The listing builds one solid part. Answer for the finished solid, in the listing's coordinates (mm). Face numbers are marked on the shaded views. A direction names the side the tool comes from. Give positions to 0.01 mm unless a question says otherwise; leave off trailing zeros. Order: outer loops, then holes, each group sorted by start corner. A loop starts at its lowest first (then second) coordinate and runs counter-clockwise, first axis right, second up. Notation, with made-up numbers: (86, 86) - (145, 86) arc R17 cw to (145, 90) - close; hole circle Ø4 at (4, 44). An arc over 180 degrees is marked (long way). Answer in a Markdown table with one row per item. Add a question column.
```python
from build123d import *

# Parameters (mm, degrees)
SKETCH3_W           = 13.5
SKETCH3_H           = 5
SKETCH3_W_2         = 10
SKETCH3_W_3         = 5
SKETCH3_H_2         = 23
BOSS_EXTRUDE1_DEPTH = 45
FILLET1_R           = 2
SKETCH5_R           = 2.1
CUT_EXTRUDE2_DEPTH  = 45
SKETCH6_R           = 2.1
CUT_EXTRUDE3_DEPTH  = 45
SKETCH7_W           = 8.210459319
SKETCH7_H           = 32.58724939
BOSS_EXTRUDE2_DEPTH = 5
SKETCH8_R           = 2.1
CUT_EXTRUDE5_DEPTH  = 45
BOSS_EXTRUDE3_DEPTH = 45
SKETCH10_W          = 60.355694637
SKETCH10_H          = 75.381613981
CUT_EXTRUDE7_DEPTH  = 9
SKETCH13_W          = 6.095088126
SKETCH13_H          = 29.055723933
BOSS_EXTRUDE6_DEPTH = 5
SKETCH14_W          = 6.424633762
SKETCH14_H          = 30.784703445
BOSS_EXTRUDE7_DEPTH = 5
FILLET3_R           = 2
SKETCH15_R          = 2.1
CUT_EXTRUDE8_DEPTH  = 9
SKETCH16_R          = 2.1
CUT_EXTRUDE9_DEPTH  = 9


with BuildPart() as part:
    # Sketch3 → Boss-Extrude1 (new body)
    with BuildSketch(Plane.XY):
        with BuildLine():
            ThreePointArc((-5.06519953, 257.264696919), (-21.146881422, 239.197551787), (-25.551614771, 215.414352888))
            Line((-25.551614771, 215.414352888), (-30.551614771, 215.414352888))
            Line((-30.551614771, 215.414352888), (-30.551614771, 220.414352888))
            ThreePointArc((-30.551614771, 220.414352888), (-24.004098535, 245.112635185), (-5.06519953, 262.264696919))
            Line((-5.06519953, 262.264696919), (-5.06519953, 257.264696919))
        make_face()
        with Locations((1.68480047, 259.764696919)):
            Rectangle(SKETCH3_W, SKETCH3_H)
        with Locations((-35.551614771, 217.914352888)):
            Rectangle(SKETCH3_W_2, SKETCH3_H)
        with Locations((-28.051614771, 203.914352888)):
            Rectangle(SKETCH3_W_3, SKETCH3_H_2)
    extrude(amount=BOSS_EXTRUDE1_DEPTH)

    # Fillet1
    fillet1_edges = [part.edges().sort_by_distance(p)[0] for p in [
        (-40.551614771, 217.914352888, 0),
        (8.43480047, 259.764696919, 45),
        (8.43480047, 259.764696919, 0),
        (-40.551614771, 217.914352888, 45),
    ]]
    fillet(fillet1_edges, radius=FILLET1_R)

    # Sketch5 → Cut-Extrude2 (cut)
    with BuildSketch(Plane(origin=(0, 262.264696919, 0), x_dir=(1, 0, 0), z_dir=(0, 1, 0))):
        with Locations((0.24480047, -40)):
            Circle(SKETCH5_R)
        with Locations((0.24480047, -14.8)):
            Circle(SKETCH5_R)
    extrude(amount=-CUT_EXTRUDE2_DEPTH, mode=Mode.SUBTRACT)

    # Sketch6 → Cut-Extrude3 (cut)
    with BuildSketch(Plane(origin=(0, 220.414352888, 0), x_dir=(1, 0, 0), z_dir=(0, 1, 0))):
        with Locations((-35.551614771, -10)):
            Circle(SKETCH6_R)
        with Locations((-35.551614771, -35)):
            Circle(SKETCH6_R)
    extrude(amount=-CUT_EXTRUDE3_DEPTH, mode=Mode.SUBTRACT)

    # Sketch7 → Boss-Extrude2 (add)
    with BuildSketch(Plane(origin=(0, 262.264696919, 0), x_dir=(1, 0, 0), z_dir=(0, 1, 0))):
        with Locations((1.09445166, -26.923464517)):
            Rectangle(SKETCH7_W, SKETCH7_H)
    extrude(amount=-BOSS_EXTRUDE2_DEPTH)

    # Sketch8 → Cut-Extrude5 (cut)
    with BuildSketch(Plane(origin=(0, 262.264696919, 0), x_dir=(1, 0, 0), z_dir=(0, 1, 0))):
        with Locations((0.24480047, -5)):
            Circle(SKETCH8_R)
        with Locations((0.24480047, -30.2)):
            Circle(SKETCH8_R)
    extrude(amount=-CUT_EXTRUDE5_DEPTH, mode=Mode.SUBTRACT)

    # Sketch9 → Boss-Extrude3 (add, through all)
    with BuildSketch(Plane.XY.offset(45)):
        with BuildLine():
            ThreePointArc((-25.265361734, 225.859750777), (-25.456525287, 224.362535182), (-25.597369426, 222.859750777))
            Line((-25.597369426, 222.859750777), (-18.597369426, 222.859750777))
            Line((-18.597369426, 222.859750777), (-15.597369426, 222.859750777))
            Line((-15.597369426, 222.859750777), (-15.597369426, 247.859750777))
            ThreePointArc((-15.597369426, 247.859750777), (-17.156118075, 245.834377519), (-18.597369426, 243.72377838))
            Line((-18.597369426, 243.72377838), (-18.597369426, 225.859750777))
            Line((-18.597369426, 225.859750777), (-25.265361734, 225.859750777))
        make_face()
        Polygon((-15.597369426, 222.859750777), (-18.597369426, 222.859750777), (-25.551614771, 215.414352888), (-25.551614771, 212.414352888), align=None)
    extrude(amount=-BOSS_EXTRUDE3_DEPTH)

    # Sketch10 → Cut-Extrude7 (cut)
    with BuildSketch(Plane.XY.offset(45)):
        with Locations((-21.743046849, 224.573889929)):
            Rectangle(SKETCH10_W, SKETCH10_H)
    extrude(amount=-CUT_EXTRUDE7_DEPTH, mode=Mode.SUBTRACT)

    # Sketch13 → Boss-Extrude6 (add)
    with BuildSketch(Plane(origin=(0, 220.414352888, 0), x_dir=(1, 0, 0), z_dir=(0, 1, 0))):
        with Locations((-35.175849568, -21.472138034)):
            Rectangle(SKETCH13_W, SKETCH13_H)
    extrude(amount=-BOSS_EXTRUDE6_DEPTH)

    # Sketch14 → Boss-Extrude7 (add)
    with BuildSketch(Plane(origin=(0, 262.264696919, 0), x_dir=(1, 0, 0), z_dir=(0, 1, 0))):
        with Locations((0.1637931, -17.411075239)):
            Rectangle(SKETCH14_W, SKETCH14_H)
    extrude(amount=-BOSS_EXTRUDE7_DEPTH)

    # Fillet3
    fillet3_edges = [part.edges().sort_by_distance(p)[0] for p in [
        (-40.551614771, 217.914352888, 36),
        (8.43480047, 259.764696919, 36),
    ]]
    fillet(fillet3_edges, radius=FILLET3_R)

    # Sketch15 → Cut-Extrude8 (cut)
    with BuildSketch(Plane(origin=(0, 220.414352888, 0), x_dir=(1, 0, 0), z_dir=(0, 1, 0))):
        with Locations((-35.551614771, -8)):
            Circle(SKETCH15_R)
        with Locations((-35.551614771, -28)):
            Circle(SKETCH15_R)
    extrude(amount=-CUT_EXTRUDE8_DEPTH, mode=Mode.SUBTRACT)

    # Sketch16 → Cut-Extrude9 (cut)
    with BuildSketch(Plane(origin=(0, 262.264696919, 0), x_dir=(1, 0, 0), z_dir=(0, 1, 0))):
        with Locations((1.68480047, -8)):
            Circle(SKETCH16_R)
        with Locations((1.68480047, -28)):
            Circle(SKETCH16_R)
    extrude(amount=-CUT_EXTRUDE9_DEPTH, mode=Mode.SUBTRACT)


solid = part.part
```
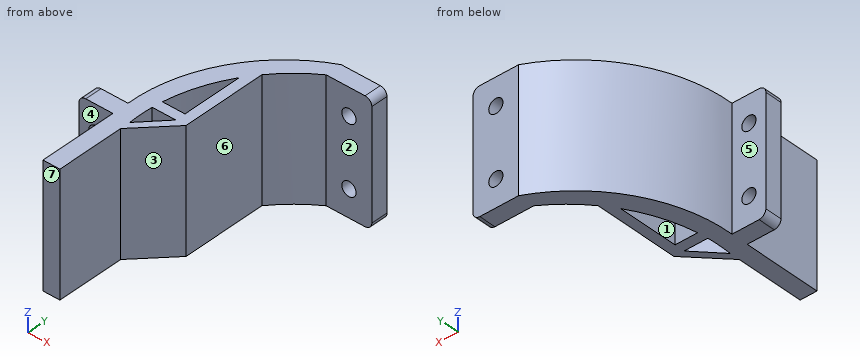
(1) Find section A-A, the plane z = 28. Write down the section's boundary in (x, y).
(2) Straight lines are drawn through the part: line 1 (X direction, y = 201.5, z = 28); line 2 (Y direction, x = -20, z = 26); line 3 (Y direction, x = -31, z = 2). For each, find the intervals that lie inside material, in ascending order.
(3) For the marked faces 4, 5, 6 and 7, determine the directions among +Z, -Z, +X, -X, +Y, -Y from which every point of the face is accessible in a straight line to the end or side of a thin tool.
(4) Find section B-B, the plane z = 3. Write down the section's boundary in (x, y).
(5) Each of these flat-tipped pins is pushed along its axis until it touches: P1, Ø2, axis at x = -20.5, z = 24, coming from the +Y side; P2, Ø3.5, axis at x = -21, z = 12, coming from the -Y side; P3, Ø5, axis at y = 207, z = 7.5, coming from the -X side; P4, Ø2.5, axis at x = 1.68, z = 28, coming from the -Y side. Where does it stop, or does it pass through?
(6) Find section C-C, the plane x = 3. Write down the section's boundary in (y, z).
(7) Find section D-D, the plane y = 205.5. Write down the section's boundary in (x, z).
(8) The mould has two halves that part along X. Classify the marked faces 1, 2 and 3: +X half, -X half, draft (parallel to the pull), parting line (faces both ways), or undercut.
Answer key:
| question | item | result |
|---|---|---|
| 1 | outline | (-40.55, 215.41) - (-37.65, 215.41) - (-37.65, 220.41) - (-40.55, 220.41) - close; (-33.45, 215.41) - (-30.55, 215.41) - (-30.55, 192.41) - (-25.55, 192.41) - (-25.55, 212.41) - (-15.6, 222.86) - (-15.6, 247.86) arc R45 cw to (-5.07, 257.26) - (-0.42, 257.26) - (-0.42, 262.26) - (-5.07, 262.26) arc R45 ccw to (-30.55, 220.41) - (-33.45, 220.41) - close; (3.78, 257.26) - (8.43, 257.26) - (8.43, 262.26) - (3.78, 262.26) - close; hole (-25.6, 222.86) arc R45 ccw to (-25.55, 215.41) - (-18.6, 222.86) - close; hole (-25.27, 225.86) - (-18.6, 225.86) - (-18.6, 243.72) arc R45 ccw to start |
| 2 | line 1 | -30.55 to -25.55 |
| 2 | line 2 | 218.24 to 221.36, 222.86 to 225.86, 241.39 to 250.68 |
| 2 | line 3 | 215.41 to 220.41 |
| 3 | face 4 | +Z, -Z, -X, -Y |
| 3 | face 5 | +Z, -Z, -X, +Y |
| 3 | face 6 | +Z, -Z, +X, -Y |
| 3 | face 7 | +Z, -Z, +X, -X, -Y |
| 4 | outline | (-40.55, 215.41) - (-30.55, 215.41) - (-30.55, 192.41) - (-25.55, 192.41) - (-25.55, 212.41) - (-15.6, 222.86) - (-15.6, 247.86) arc R45 cw to (-5.07, 257.26) - (8.43, 257.26) - (8.43, 262.26) - (-5.07, 262.26) arc R45 ccw to (-30.55, 220.41) - (-40.55, 220.41) - close; hole (-25.6, 222.86) arc R45 ccw to (-25.55, 215.41) - (-18.6, 222.86) - close; hole (-25.27, 225.86) - (-18.6, 225.86) - (-18.6, 243.72) arc R45 ccw to start |
| 5 | P1 | y = 251.27 |
| 5 | P2 | y = 215.35 |
| 5 | P3 | x = -30.55 |
| 5 | P4 | through |
| 6 | outline | (257.26, 0) - (262.26, 0) - (262.26, 6.36) - (257.26, 6.36) - close; (257.26, 9.64) - (262.26, 9.64) - (262.26, 26.36) - (257.26, 26.36) - close; (257.26, 29.64) - (262.26, 29.64) - (262.26, 36) - (257.26, 36) - close |
| 7 | outline | (-30.55, 0) - (-25.55, 0) - (-25.55, 36) - (-30.55, 36) - close |
| 8 | face 1 | undercut |
| 8 | face 2 | draft |
| 8 | face 3 | +X half |
